Check sheet for the modelled part. Datum: model origin and axes. Units: mm. A direction names the side the tool comes from. Coordinates: 2 decimals unless noted, no trailing zeros. Loops run counter-clockwise (first coordinate to the right, second up) from the corner with the lowest first, then second, coordinate; pieces in that order, holes last. Notation, with made-up numbers: M 4.5,42 L 41.5,42 A24 ccw 41.5,52 Z; hole C 32,45.25 d7. An arc over 180 degrees is marked long. Answer as CSV lines item,"result". Start each with the question number.
from build123d import *

# Parameters (mm, degrees)
SKETCH1_W            = 40.5
SKETCH1_H            = 20
BOSS_EXTRUDE1_DEPTH  = 35.5
BOSS_EXTRUDE2_DEPTH  = 2
SKETCH3_R            = 6.4
BOSS_EXTRUDE3_DEPTH  = 1
SKETCH4_R            = 5.575
BOSS_EXTRUDE4_DEPTH  = 0.5
BOSS_EXTRUDE5_DEPTH  = 2.5
MIRROR2_COPY_1_DEPTH = 2.5
CHAMFER1_SIZE        = 1
SKETCH6_W            = 3
SKETCH6_H            = 1
BOSS_EXTRUDE6_DEPTH  = 6
DRAFT1_ANGLE         = 10
SKETCH7_W            = 14.691761142
SKETCH7_H            = 18
SKETCH7_W_2          = 13.691761142
SKETCH7_H_2          = 17
BOSS_EXTRUDE7_DEPTH  = 0.5


with BuildPart() as part:
    # Sketch1 → Boss-Extrude1 (new body)
    with BuildSketch(Plane(origin=(0, 0, 0), x_dir=(1, 0, 0), z_dir=(0, 1, 0))):
        Rectangle(SKETCH1_W, SKETCH1_H)
    extrude(amount=BOSS_EXTRUDE1_DEPTH)

    # Sketch2 → Boss-Extrude2 (add)
    with BuildSketch(Plane(origin=(0, 35.5, 0), x_dir=(1, 0, 0), z_dir=(0, 1, 0))):
        with BuildLine():
            Line((-5.75, -9), (14.25, -9))
            Line((14.25, -9), (14.25, -4.8))
            ThreePointArc((14.25, -4.8), (16.65, 0), (14.25, 4.8))
            Line((14.25, 4.8), (14.25, 9))
            Line((14.25, 9), (-5.75, 9))
            ThreePointArc((-5.75, 9), (-20.108898944, 0), (-5.75, -9))
        make_face()
    extrude(amount=BOSS_EXTRUDE2_DEPTH)

    # Sketch3 → Boss-Extrude3 (add)
    with BuildSketch(Plane(origin=(0, 37.5, 0), x_dir=(1, 0, 0), z_dir=(0, 1, 0))):
        with Locations(Location((-10.108898944, 0, 0), (0, 0, 270))):
            Circle(SKETCH3_R)
    extrude(amount=BOSS_EXTRUDE3_DEPTH)

    # Sketch4 → Boss-Extrude4 (add)
    with BuildSketch(Plane(origin=(0, 38.5, 0), x_dir=(1, 0, 0), z_dir=(0, 1, 0))):
        with Locations(Location((-10.108898944, 0, 0), (0, 0, 270))):
            Circle(SKETCH4_R)
    extrude(amount=BOSS_EXTRUDE4_DEPTH)

    # Sketch5 → Boss-Extrude5 (add)
    with BuildSketch(Plane(origin=(0, 29.5, 0), x_dir=(1, 0, 0), z_dir=(0, 1, 0))):
        with BuildLine():
            Line((20.25, 9), (27.25, 9))
            Line((27.25, 9), (27.25, 6.25))
            Line((27.25, 6.25), (26.177050983, 6.25))
            ThreePointArc((26.177050983, 6.25), (22.25, 4.75), (26.177050983, 3.25))
            Line((26.177050983, 3.25), (27.25, 3.25))
            Line((27.25, 3.25), (27.25, 0))
            Line((27.25, 0), (20.25, 0))
            Line((20.25, 0), (20.25, 9))
        make_face()
    boss_extrude5 = extrude(amount=-BOSS_EXTRUDE5_DEPTH)

    # Mirror1: Boss-Extrude5 across plane
    add(boss_extrude5.mirror(Plane(origin=(0, 0, 0), x_dir=(0, 0, 1), z_dir=(1, 0, 0))))

    # Mirror2: Boss-Extrude5 across plane
    add(boss_extrude5.mirror(Plane.XY))

    # Mirror2 copy 1 sketch → Mirror2 copy 1 (add)
    with BuildSketch(Plane(origin=(0, 29.5, 0), x_dir=(-1, 0, 0), z_dir=(0, 1, 0))):
        with BuildLine():
            Line((20.25, 9), (27.25, 9))
            Line((27.25, 9), (27.25, 6.25))
            Line((27.25, 6.25), (26.177050983, 6.25))
            ThreePointArc((26.177050983, 6.25), (22.25, 4.75), (26.177050983, 3.25))
            Line((26.177050983, 3.25), (27.25, 3.25))
            Line((27.25, 3.25), (27.25, 0))
            Line((27.25, 0), (20.25, 0))
            Line((20.25, 0), (20.25, 9))
        make_face()
    extrude(amount=-MIRROR2_COPY_1_DEPTH)

    # Chamfer1
    chamfer1_edges = [part.edges().sort_by_distance(p)[0] for p in [
        (0, 0, -10),
        (20.25, 0, 0),
        (0, 0, 10),
        (-20.25, 0, 0),
    ]]
    chamfer(chamfer1_edges, length=CHAMFER1_SIZE)

    # Sketch6 → Boss-Extrude6 (add)
    with BuildSketch(Plane.ZY.offset(20.25)):
        with Locations((0, 3)):
            Rectangle(SKETCH6_W, SKETCH6_H)
    extrude(amount=BOSS_EXTRUDE6_DEPTH)

    # Draft1
    draft1_faces = [part.faces().sort_by_distance(p)[0] for p in [
        (-23.25, 3, -1.5),
        (-23.25, 3.5, 0),
        (-23.25, 3, 1.5),
        (-23.25, 2.5, 0),
    ]]
    draft(draft1_faces, Plane(origin=(-26.25, 0, 0), x_dir=(0, 0, -1), z_dir=(-1, 0, 0)), DRAFT1_ANGLE)

    # Sketch7 → Boss-Extrude7 (add)
    with BuildSketch(Plane(origin=(0, 37.5, 0), x_dir=(1, 0, 0), z_dir=(0, 1, 0))):
        with Locations((6.904119429, 0)):
            Rectangle(SKETCH7_W, SKETCH7_H)
        with Locations((6.904119429, 0)):
            Rectangle(SKETCH7_W_2, SKETCH7_H_2, mode=Mode.SUBTRACT)
    extrude(amount=BOSS_EXTRUDE7_DEPTH)


solid = part.part
Item 1: Sectioned sample at B-B, the plane x = 3.5. Record the boundary of the cut face in (y, z).
Item 2: Sectioned sample at C-C, the plane x = -24.5. Record the boundary of the cut face in (y, z), and give its area (3 significant figures).
Item 3: Go/stop test with flat-tipped pins: pin 1 (1 mm diameter, centred on y = 8, z = -2.5, fed in from -X); pin 2 (4 mm diameter, centred on x = 5.5, z = 7, fed in from +Y); pin 3 (2 mm diameter, centred on x = -23, z = -3.5, fed in from +Y). Record where each tip stops, or that it passes through.
Item 4: Material ranges on line 1 (Z direction, x = -24.5, y = 28.4); line 2 (X direction, y = 21, z = 6.5); line 3 (Y direction, x = -1, z = -5.5), recorded low to high. Write a range as from..to.
Item 5: Sectioned sample at A-A, the plane x = 24.5. Record the boundary of the cut face in (y, z).
Item 6: Set-up check for faces 4 (the face through (-20.09, 35.5, 2.18)), 5 (the face through (-27, 28, -6.25)), 6 (the face through (-23.208, 4.036, -0.036)): record each of +Z, -Z, +X, -X, +Y, -Y from which the full face is reachable in a straight line by a thin tool's end or side.
Item 7: Release check for a two-part mould opening along Z. For faces 1 (the face through (-27, 28, 3.25)), 2 (the face through (20.25, 18, 0)), 3 (the face through (4, 37, 9)) record: released by +Z, released by -Z, zero draft, split by the parting line, or undercut.
Reply:
1,outline,"M 0,-9 L 1,-10 L 35.5,-10 L 35.5,-9 L 38,-9 L 38,-8.5 L 37.5,-8.5 L 37.5,8.5 L 38,8.5 L 38,9 L 35.5,9 L 35.5,10 L 1,10 L 0,9 Z"
2,outline,"M 2.19,-1.81 L 3.81,-1.81 L 3.81,1.81 L 2.19,1.81 Z; M 27,-9 L 29.5,-9 L 29.5,-7 L 27,-7 Z; M 27,-2.5 L 29.5,-2.5 L 29.5,2.5 L 27,2.5 Z; M 27,7 L 29.5,7 L 29.5,9 L 27,9 Z"
2,area,"28.3 mm²"
3,pin 1,"x = -20.25"
3,pin 2,"y = 38"
3,pin 3,"y = 29.5"
4,line 1,"-9..-7, -2.5..2.5, 7..9"
4,line 2,"-20.25..20.25"
4,line 3,"0..37.5"
5,outline,"M 27,-9 L 29.5,-9 L 29.5,-7 L 27,-7 Z; M 27,-2.5 L 29.5,-2.5 L 29.5,2.5 L 27,2.5 Z; M 27,7 L 29.5,7 L 29.5,9 L 27,9 Z"
6,face 4,"-X, +Y"
6,face 5,"-X, +Y, -Y"
6,face 6,"+Z, -Z, -X"
7,face 1,"undercut"
7,face 2,"zero draft"
7,face 3,"released by +Z"
